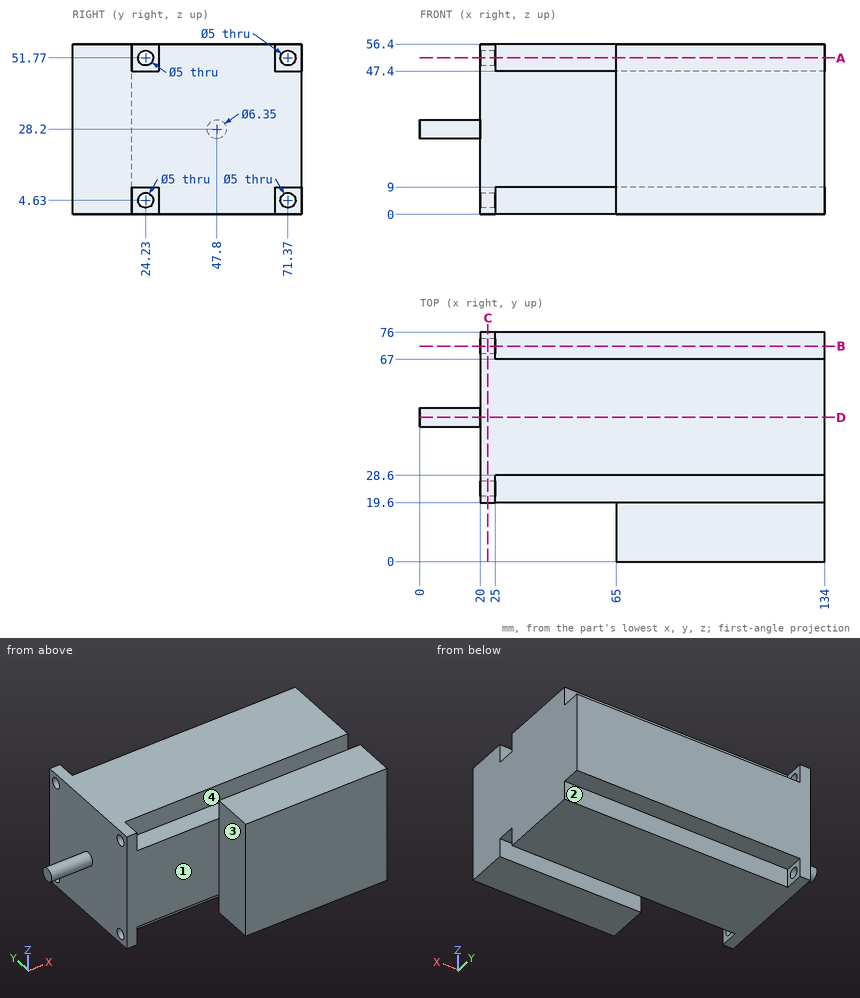
Can you work these out from the drawing? Everything is in mm from the part's minimum corner. Give positions to 0.01 mm unless a question says otherwise; leave off trailing zeros. Loops run counter-clockwise (first coordinate to the right, second up) from the corner with the lowest first, then second, coordinate; pieces in that order, holes last. Notation, with made-up numbers: M 6,37.5 L 24,37.5 A14 cw 24,59.5 Z; hole C 69.25,-35.75 d7. An arc over 180 degrees is marked long. Put each result on its own line as item: value. Start each with the question number.
(1) I want a section at A-A on z = 51.77. Please give me the cut outline in (x, y), then the cut area to 3 significant figures.
(2) Will these pins go through, and if not, where does the flat tip stop? pin 1 Ø5 at (y, z) = (36.5, 50.5) entering from -X; pin 2 Ø4.5 at (y, z) = (24, 54) entering from +X; pin 3 Ø7 at (x, y) = (55, 73.5) entering from -Z; pin 4 Ø4.5 at (y, z) = (71.37, 51.77) entering from +X.
(3) I want a section at D-D on y = 47.8. Please give me the cut outline in (x, z) (3 decimals), then the cut area to 3 significant figures.
(4) I want a section at B-B on y = 71.37. Please give me the cut outline in (x, z).
(5) If we mould it in two halves opening along Y, with no side actions, what happens to the marked faces 1, 2, 3 and 4? For each: +Y half, -Y half, draft (parallel to the pull), parting line (faces both ways), or undercut.
(6) I need wall thicknesses on line 1 along Y through (x, z) = (21.1, 4.63); line 2 along Y through (x, z) = (22, 4); line 3 along X through (y, z) = (66, 13.5). Which ranges of each line are inside material? Lowest first, please. Write a range as [from, to].
(7) I want a section at C-C on x = 22.5. Please give me the cut outline in (y, z), then the cut area to 3 significant figures.
Answer block:
1. outline: M 20,19.6 L 25,19.6 L 25,21.73 L 20,21.73 Z; M 20,26.73 L 25,26.73 L 25,28.6 L 134,28.6 L 134,67 L 25,67 L 25,68.87 L 20,68.87 Z; M 20,73.87 L 25,73.87 L 25,76 L 20,76 Z; M 65,0 L 134,0 L 134,19.6 L 65,19.6 Z
1. area: 5,770 mm^2
2. pin 1: x = 20
2. pin 2: x = 25
2. pin 3: z = 9
2. pin 4: through
3. outline: M 0,25.025 L 20,25.025 L 20,0 L 134,0 L 134,56.4 L 20,56.4 L 20,31.375 L 0,31.375 Z
3. area: 6,560 mm^2
4. outline: M 20,0 L 25,0 L 25,2.13 L 20,2.13 Z; M 20,7.13 L 25,7.13 L 25,9 L 134,9 L 134,47.4 L 25,47.4 L 25,49.27 L 20,49.27 Z; M 20,54.27 L 25,54.27 L 25,56.4 L 20,56.4 Z
5. face 1: -Y half
5. face 2: +Y half
5. face 3: draft
5. face 4: undercut
6. line 1: [19.6, 21.73], [26.73, 68.87], [73.87, 76]
6. line 2: [19.6, 21.81], [26.65, 68.95], [73.79, 76]
6. line 3: [20, 134]
7. outline: M 19.6,0 L 76,0 L 76,56.4 L 19.6,56.4 Z; hole C 24.23,4.63 d5; hole C 24.23,51.77 d5; hole C 71.37,4.63 d5; hole C 71.37,51.77 d5
7. area: 3,100 mm^2
